Input: dimensioned drawing with shaded views. Units: mm. Origin: part minimum x, y, z. Coordinates: 2 decimals unless noted, no trailing zeros. Order: outer loops, then holes, each group sorted by start corner. A loop starts at its lowest first (then second) coordinate and runs counter-clockwise, first axis right, second up. Notation, with made-up numbers: (-38, 57.25) -> (-3, 57.25) arc R17 ccw to (-3, 71.25) -> close; hole circle Ø3 at (-23.5, 37). An arc over 180 degrees is marked (long way). Write item = value, one per line. Start each with the question number.
Item 1: Section query C-C (z = 69.2). Output: boundary loops of the cut face in (x, y).
Item 2: Section query B-B (y = 4.75). Output: boundary loops of the cut face in (x, z) (1 decimal), then the cut area to 3 significant figures.
Item 3: Section query D-D (x = 35). Output: boundary loops of the cut face in (y, z).
Item 4: Contact query for a flat-ended pin moving along its axis: pin 1 (1.5 mm diameter, centred on x = 13.5, y = 3, fed in from -Z). Output: stop coordinate, or through.
Item 5: Ray query, line 1 along X through (y, z) = (3, 10); line 2 along X through (y, z) = (5.5, 69.2); line 3 along Z through (x, y) = (9, 2). Return the intervals inside material, ascending. Write a range as [from, to].
Item 6: Section query A-A (x = 20). Output: boundary loops of the cut face in (y, z).
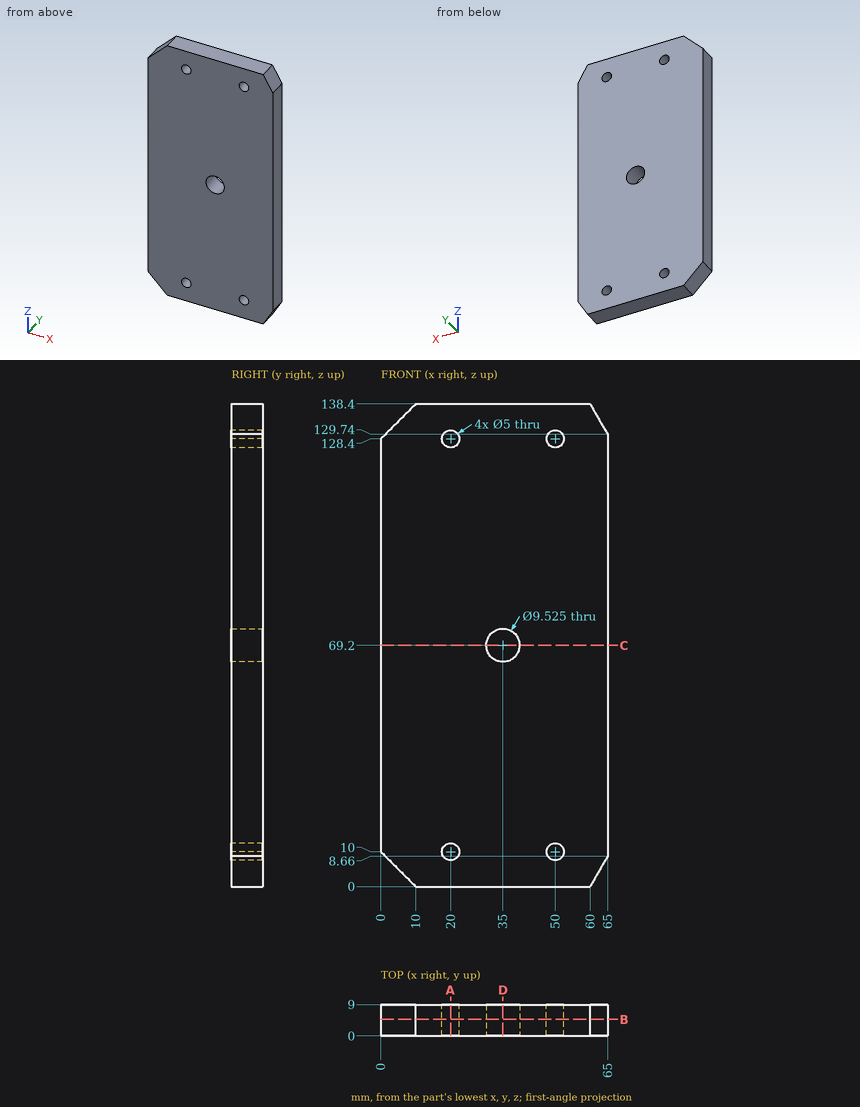
Computed:
q1.outline = (0, 0) -> (30.24, 0) -> (30.24, 9) -> (0, 9) -> close; (39.76, 0) -> (65, 0) -> (65, 9) -> (39.76, 9) -> close
q2.outline = (0, 10) -> (10, 0) -> (60, 0) -> (65, 8.7) -> (65, 129.7) -> (60, 138.4) -> (10, 138.4) -> (0, 128.4) -> close; hole circle Ø5 at (20, 10); hole circle Ø5 at (20, 128.4); hole circle Ø9.5 at (35, 69.2); hole circle Ø5 at (50, 10); hole circle Ø5 at (50, 128.4)
q2.area = 8,700 mm^2
q3.outline = (0, 0) -> (9, 0) -> (9, 64.44) -> (0, 64.44) -> close; (0, 73.96) -> (9, 73.96) -> (9, 138.4) -> (0, 138.4) -> close
q4.pin_1 = 0
q5.line_1 = [0, 17.5], [22.5, 47.5], [52.5, 65]
q5.line_2 = [0, 30.24], [39.76, 65]
q5.line_3 = [1, 137.4]
q6.outline = (0, 0) -> (9, 0) -> (9, 7.5) -> (0, 7.5) -> close; (0, 12.5) -> (9, 12.5) -> (9, 125.9) -> (0, 125.9) -> close; (0, 130.9) -> (9, 130.9) -> (9, 138.4) -> (0, 138.4) -> close
